Read the model definition and answer for the solid it produces. Units are mm, in the model's axes. Face numbers are marked on the shaded views. A direction names the side the tool comes from. Coordinates: 2 decimals unless noted, no trailing zeros. Loops run counter-clockwise (first coordinate to the right, second up) from the corner with the lowest first, then second, coordinate; pieces in that order, holes last. Notation, with made-up numbers: (23, 62.5) -> (34, 62.5) arc R35 cw to (34, 96.5) -> close; hole circle Ø3 at (-14, 58.5). An arc over 180 degrees is marked (long way). Answer in a Markdown table with one row per item.
```python
from build123d import *

# Parameters (mm, degrees)
SKETCH1_R                              = 22.225
BOSS_EXTRUDE1_DEPTH                    = 50.8
SKETCH2_OUTSIDE_W                      = 62.614
SKETCH2_OUTSIDE_H                      = 62.614
SKETCH2_OUTSIDE_R                      = 7.9375
CUT_EXTRUDE1_DEPTH                     = 31.75
F_1_8_0_125_DIAMETER_HOLE1_D           = 3.175
F_1_8_START                            = -22.225000076
F_1_8_0_125_DIAMETER_HOLE2_OUTLINE_R   = 1.5875
F_1_8_0_125_DIAMETER_HOLE2_DEPTH       = 31.186397695
F_1_8_START_2                          = -8.961397619
F_1_8_0_125_DIAMETER_HOLE2_2_OUTLINE_R = 1.5875
F_1_8_0_125_DIAMETER_HOLE2_2_DEPTH     = 17.922795238
F_1_8_27_NPSM_TAPPED_HOLE1_D           = 9.0932
F_1_8_27_NPSM_TAPPED_HOLE1_DEPTH       = 6.35
F_1_8_27_NPSM_TAPPED_HOLE1_TIP         = 2.73187289
CUT_EXTRUDE2_START                     = -13.97
SKETCH11_R                             = 4.5466
CUT_EXTRUDE2_DEPTH                     = 6.35
SKETCH12_R                             = 2.54
CUT_EXTRUDE3_DEPTH                     = 1.5875
CUT_EXTRUDE5_START                     = -31.75
SKETCH13_OUTSIDE_W                     = 62.614
SKETCH13_OUTSIDE_H                     = 62.614
SKETCH13_OUTSIDE_R                     = 6.35
CUT_EXTRUDE5_DEPTH                     = 1.5875


# Read off the part's stored shape, not the designer's step: 1/8 (0.125) Diameter Hole2
with BuildPart() as part:
    # Sketch1 → Boss-Extrude1 (new body)
    with BuildSketch(Plane(origin=(0, 0, 0), x_dir=(1, 0, 0), z_dir=(0, 1, 0))):
        with Locations(Location((0, 0, 0), (0, 0, 270))):
            Circle(SKETCH1_R)
    extrude(amount=BOSS_EXTRUDE1_DEPTH)

    # Sketch2 outside → Cut-Extrude1 (cut)
    with BuildSketch(Plane(origin=(0, 0, 0), x_dir=(-1, 0, 0), z_dir=(0, -1, 0))):
        Rectangle(SKETCH2_OUTSIDE_W, SKETCH2_OUTSIDE_H)
        with Locations(Location((0, 0, 0), (0, 0, 90))):
            Circle(SKETCH2_OUTSIDE_R, mode=Mode.SUBTRACT)
    extrude(amount=-CUT_EXTRUDE1_DEPTH, mode=Mode.SUBTRACT)

    # 1/8 (0.125) Diameter Hole1 (through all)
    with Locations(Plane(origin=(0, 50.8, 0), x_dir=(1, 0, 0), z_dir=(0, 1, 0))):
        with Locations((0, 0)):
            Hole(F_1_8_0_125_DIAMETER_HOLE1_D / 2)

    # Sketch6 → 1/4 NPT Tapped Hole1 (revolve, cut)
    with BuildSketch(Plane(origin=(0, 50.8, 0), x_dir=(0, 0, 1), z_dir=(1, 0, 0))):
        Polygon((0, 0), (0, 20.275689079), (5.5626, 16.9333418), (5.5626, 9.906), (6.557984794, 9.906), (6.8545837, 0), align=None)
    revolve(axis=Axis((0, 57.15, 0), (0, -1, 0)), mode=Mode.SUBTRACT)

    # Sketch8 → 1/8 NPT Tapped Hole1 (revolve, cut)
    with BuildSketch(Plane(origin=(22.225, 41.275, 0), x_dir=(0, 0, -1), z_dir=(0, 1, 0))):
        Polygon((0, 0), (0, 14.217468714), (4.2164, 11.684), (4.2164, 6.858), (4.936181096, 6.858), (5.1415188, 0), align=None)
    revolve(axis=Axis((28.575, 41.275, 0), (-1, 0, 0)), mode=Mode.SUBTRACT)

    # Sketch8 at point 2 (carried to point 2, square into its face) → 1/8 NPT Tapped Hole1 at 2 (revolve, cut)
    with BuildSketch(Plane(origin=(0, 41.275, -22.225), x_dir=(-1, 0, 0), z_dir=(0, 1, 0))):
        Polygon((0, 0), (0, 14.217468714), (4.2164, 11.684), (4.2164, 6.858), (4.936181096, 6.858), (5.1415188, 0), align=None)
    revolve(axis=Axis((0, 41.275, -28.575), (0, 0, 1)), mode=Mode.SUBTRACT)

    # Sketch8 at point 3 (carried to point 3, square into its face) → 1/8 NPT Tapped Hole1 at 3 (revolve, cut)
    with BuildSketch(Plane(origin=(0, 41.275, 22.225), x_dir=(1, 0, 0), z_dir=(0, 1, 0))):
        Polygon((0, 0), (0, 14.217468714), (4.2164, 11.684), (4.2164, 6.858), (4.936181096, 6.858), (5.1415188, 0), align=None)
    revolve(axis=Axis((0, 41.275, 28.575), (0, 0, -1)), mode=Mode.SUBTRACT)

    # 1/8 (0.125) Diameter Hole2 outline → 1/8 (0.125) Diameter Hole2 (cut)
    with BuildSketch(Plane.YZ.offset(F_1_8_START)):
        with Locations((41.275, 0)):
            Circle(F_1_8_0_125_DIAMETER_HOLE2_OUTLINE_R)
    extrude(amount=F_1_8_0_125_DIAMETER_HOLE2_DEPTH, mode=Mode.SUBTRACT)

    # 1_8 _0.125_ Diameter Hole2 2 outline → 1_8 _0.125_ Diameter Hole2 2 (cut)
    with BuildSketch(Plane.XY.offset(F_1_8_START_2)):
        with Locations((0, 41.275)):
            Circle(F_1_8_0_125_DIAMETER_HOLE2_2_OUTLINE_R)
    extrude(amount=F_1_8_0_125_DIAMETER_HOLE2_2_DEPTH, mode=Mode.SUBTRACT)

    # 1/8-27 NPSM Tapped Hole1
    with Locations(Plane(origin=(-22.225, 41.275, 0), x_dir=(0, 0, -1), z_dir=(-1, 0, 0))):
        with Locations((0, 0)):
            Hole(F_1_8_27_NPSM_TAPPED_HOLE1_D / 2, depth=F_1_8_27_NPSM_TAPPED_HOLE1_DEPTH)
            with Locations((0, 0, -(F_1_8_27_NPSM_TAPPED_HOLE1_DEPTH + F_1_8_27_NPSM_TAPPED_HOLE1_TIP / 2))):  # 118° drill point
                Cone(0, F_1_8_27_NPSM_TAPPED_HOLE1_D / 2, F_1_8_27_NPSM_TAPPED_HOLE1_TIP, mode=Mode.SUBTRACT)

    # Sketch11 → Cut-Extrude2 (cut)
    with BuildSketch(Plane(origin=(0, 0, 0), x_dir=(0, 0, -1), z_dir=(1, 0, 0)).offset(CUT_EXTRUDE2_START)):
        with Locations(Location((0, 41.275, 0), (0, 0, 180))):
            Circle(SKETCH11_R)
    extrude(amount=-CUT_EXTRUDE2_DEPTH, mode=Mode.SUBTRACT)

    # Sketch12 → Cut-Extrude3 (cut)
    with BuildSketch(Plane.ZY.offset(13.97)):
        with Locations((0, 41.275)):
            Circle(SKETCH12_R)
    extrude(amount=-CUT_EXTRUDE3_DEPTH, mode=Mode.SUBTRACT)

    # Sketch13 outside → Cut-Extrude5 (cut)
    with BuildSketch(Plane.XZ.offset(CUT_EXTRUDE5_START)):
        Rectangle(SKETCH13_OUTSIDE_W, SKETCH13_OUTSIDE_H)
        with Locations(Location((0, 0, 0), (0, 0, 270))):
            Circle(SKETCH13_OUTSIDE_R, mode=Mode.SUBTRACT)
    extrude(amount=CUT_EXTRUDE5_DEPTH, mode=Mode.SUBTRACT)


solid = part.part
```
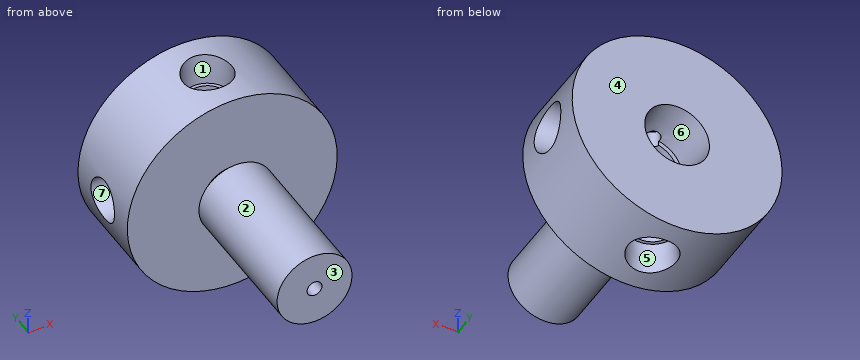
1. A cutting plane is placed at C-C on x = 18.5. Give the vertices of the cut face in (y, z) (3 decimals).
A:
| item | result |
|---|---|
| outline | (31.75, -12.317) -> (50.8, -12.317) -> (50.8, 12.317) -> (31.75, 12.317) -> close; hole circle Ø10.06 at (41.275, 0) |
2. A cutting plane is placed at D-D on x = 0. Count the separate pieces of the cut face and the enclosed holes in it, and give its area (3 significant figures).
A:
| item | result |
|---|---|
| separate pieces | 4 |
| enclosed holes | 0 |
| area | 762 mm2 |
3. A cutting plane is placed at B-B on y = 20. Give the vertices of the cut face in (x, z) (1 decimal), and give its area (3 significant figures).
A:
| item | result |
|---|---|
| outline | circle Ø15.9 at (0, 0); hole circle Ø3.2 at (0, 0) |
| area | 190 mm2 |
4. A tool of negligible diameter and unlimited length cuts with its end or side. For the marked faces 5, 6 and 7, from which of +Z, -Z, +X, -X, +Y, -Y can it reach the whole face along a straight path? Write none if from no direction.
A:
| item | result |
|---|---|
| face 5 | -Z |
| face 6 | +Y |
| face 7 | -X |
5. Given pin 1 Ø5 at (x, z) = (0, 0) entering from +Y; pin 2 Ø6.5 at (y, z) = (41.275, 0) entering from -X; pin 3 Ø1.4 at (x, z) = (-4.5, -3) entering from +Y, each flat-ended and moving along its own axis, determine where each tip first touches the part or whether it passes through.
A:
| item | result |
|---|---|
| pin 1 | stops at y = 32.03 |
| pin 2 | stops at x = -13.97 |
| pin 3 | stops at y = 40.89 |
6. Find the intervals of material crossed by probe 1 along Y at (x, z) = (7.45, 0); probe 2 along Y at (x, z) = (13.8, 0); probe 3 along Y at (x, z) = (-12, -17), in increasing order.
A:
| item | result |
|---|---|
| probe 1 | y = 0 to 30.16, 31.75 to 39.69, 42.86 to 50.8 |
| probe 2 | y = 31.75 to 37.06, 45.49 to 50.8 |
| probe 3 | y = 31.75 to 50.8 |
7. A cutting plane is placed at A-A on z = 18. Give the vertices of the cut face in (x, y) (3 decimals).
A:
| item | result |
|---|---|
| outline | (-13.037, 31.75) -> (13.037, 31.75) -> (13.037, 50.8) -> (-13.037, 50.8) -> close; hole circle Ø10.03 at (0, 41.275) |
8. The mould has two halves that part along Y. Classify the marked faces 1, 2, 3 and 4: pulls with the +Y half, pulls with the -Y half, needs draft (parallel to the pull), parting line crosses it, or undercut.
A:
| item | result |
|---|---|
| face 1 | undercut |
| face 2 | needs draft |
| face 3 | pulls with the -Y half |
| face 4 | pulls with the +Y half |
